Autodesk Inventor part; units mm, degrees
ref_plane "Work Plane3" through (1.5, 0, 13) normal (1, 0, 0) x (0, 0, -1)
ref_plane "Work Plane5" through (3, 0, 0) normal (0, 0, 1) x (0, 1, 0)
ref_plane "Work Plane6" through (0, 1.1, 0) normal (0, -1, 0) x (1, 0, 0)
sketch "Sketch1" plane through (0, 0, 0) normal (0, 1, 0) x (-1, 0, 0)
  line L0 (0, 0) -> (0, -5)
  line L1 (0, 0) -> (0, 5)
  line L2 (0, 5) -> (-3, 5)
  line L3 (0, -5) -> (-3, -5)
  line L4 (-3, 5) -> (-3, 13)
  line L5 (-3, -5) -> (-3, -13)
  line L6 (1.5, 0) -> (1.5, -5)
  line L7 (1.5, 0) -> (1.5, 5)
  spline S0 degree 3 poles (-3, 13) (1.5, 11.5121) (1.5, 8.2561) (1.5, 5) knots 0 0 0 0 1 1 1 1
  spline S1 degree 3 poles (-3, -13) (1.5, -11.5121) (1.5, -8.2561) (1.5, -5) knots 0 0 0 0 1 1 1 1
  point P0 (-3, 9)
  point P1 (-3, -9)
  dimension "d0" = 5
  dimension "d1" = 5
  dimension "d2" = 3
  dimension "d3" = 3
  dimension "d4" = 8
  dimension "d5" = 8
  dimension "d6" = 5
  dimension "d7" = 5
extrude "Extrusion1" add sketch "Sketch1" along normal blind 5
sketch "Sketch2" plane through (3, 0, 13) normal (1, 0, 0) x (0, 0, -1)
  circle A0 centre (3.5513, 2.5007) radius 1
  line L0 (13, 0) -> (13, 5)
  line L1 (8, 5) -> (18, 5)
  line L2 (4.7093, 4.4988) -> (5.8606, 2.4969)
  line L3 (5.8606, 2.4969) -> (4.7026, 0.4988)
  line L4 (4.7026, 0.4988) -> (2.3933, 0.5026)
  line L5 (2.3933, 0.5026) -> (1.2419, 2.5045)
  line L6 (1.2419, 2.5045) -> (2.3999, 4.5026)
  line L7 (2.3999, 4.5026) -> (4.7093, 4.4988)
  point P0 (22, 2.5)
  dimension "d12" = 2
  dimension "d33" = 4
extrude "Extrusion2" cut sketch "Sketch2" against normal blind 2 contours A0
ref_plane "Work Plane3" through (1.5, 0, 13) normal (1, 0, 0) x (0, 0, -1)
sketch "Sketch3" plane through (1.5, 0, 13) normal (1, 0, 0) x (0, 0, -1)
  circle A0 centre (3.5513, 2.5007) radius 1
  circle A1 centre (3.5513, 2.5007) radius 1
  line L0 (0, 0) -> (8, 0)
  line L1 (8, 0) -> (8, 5)
  line L2 (0, 5) -> (8, 5)
  line L3 (0, 0) -> (0, 5)
  line L4 (2.3935, 0.5024) -> (1.2419, 2.5042)
  line L5 (1.2419, 2.5042) -> (2.3996, 4.5024)
  line L6 (2.3996, 4.5024) -> (4.709, 4.4989)
  line L7 (4.709, 4.4989) -> (5.8607, 2.4972)
  line L8 (5.8607, 2.4972) -> (4.7029, 0.4989)
  line L9 (4.7029, 0.4989) -> (2.3935, 0.5024)
  circle A2 centre (3.5513, 2.5007) radius 1
  point P0 (13, 0)
extrude "Extrusion3" cut sketch "Sketch3" against normal blind 10 contours A0 | L4 L5 L6 L7 L8 L9
ref_plane "Work Plane5" through (3, 0, 0) normal (0, 0, 1) x (0, 1, 0)
mirror "Mirror1" about plane through (3, 0, 0) normal (0, 0, 1) of "Extrusion2", "Extrusion3"
ref_plane "Work Plane6" through (0, 1.1, 0) normal (0, -1, 0) x (1, 0, 0)
sketch "Sketch5" plane through (0, 1.1, 0) normal (0, -1, 0) x (1, 0, 0)
  line L0 (3, 5) -> (0, 5)
  line L1 (0, 5) -> (0, -5)
  line L2 (1, 5) -> (0, 4)
  line L3 (0, -5) -> (3, -5)
  line L4 (1, -5) -> (0, -4)
  point P0 (0, 0)
extrude "Extrusion4" add sketch "Sketch5" against normal blind 0.5
ref_plane "Work Plane7" through (0, 4.9, 0) normal (0, 1, 0) x (1, 0, 0)
sketch "Sketch6" plane through (0, 4.9, 0) normal (0, 1, 0) x (1, 0, 0)
  line L0 (1, -5) -> (0, -5)
  line L1 (1, -5) -> (0, -4)
  line L2 (0, -5) -> (0, -4)
  line L3 (0, 4) -> (0, 5)
  line L4 (0, 4) -> (1, 5)
  line L5 (0, 5) -> (1, 5)
  point P0 (0, 0)
extrude "Extrusion5" add sketch "Sketch6" against normal blind 0.5
properties part number "top_mount"
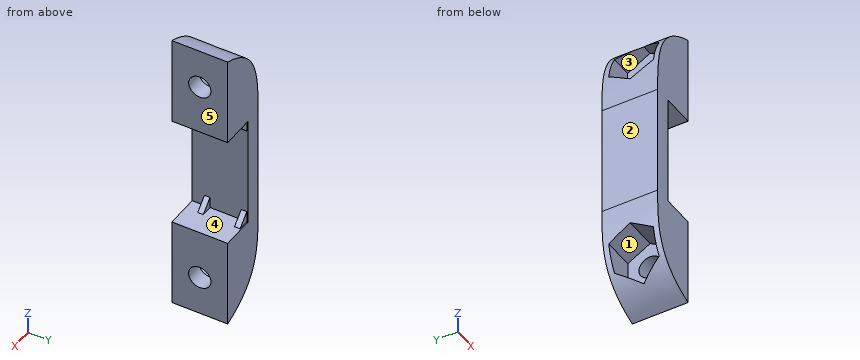
Can you work these out from the model? Positions are in its coordinate system, mm. Face numbers are marked on the shaded views. A direction names the side the tool comes from. Round coordinates to 2 decimals unless told otherwise and drop trailing zeros. Order: outer loops, then holes, each group sorted by start corner. A loop starts at its lowest first (then second) coordinate and runs counter-clockwise, first axis right, second up.
(1) If we section it at A-A (z = 2.25): Please give me the cut outline in (x, y).
Results are:
outline: (-1.5, 0) - (0, 0) - (0, 5) - (-1.5, 5) - close
(2) We'd pull the mould along Z, two halves only. Please class the marked faces 1 and 2: +Z half, -Z half, draft (parallel to the pull), parting line (faces both ways), or undercut.
Results are:
face 1: undercut
face 2: draft
(3) I'm going to push flat-ended pins straight in: pin 1 (2.5 mm diameter, centred on y = 3.5, z = 0, fed in from +X); pin 2 (1.5 mm diameter, centred on x = 2, y = 1.5, fed in from +Z); pin 3 (1.5 mm diameter, centred on y = 2, z = -8, fed in from -X). Where does each tip first touch, or does it pass through?
Results are:
pin 1: stops at x = 0
pin 2: stops at z = 12.91
pin 3: stops at x = -1.44
(4) If I drill on L1, parallel to Z at x = 2.45, y = 2; L2, parallel to Y at x = -0.45, z = 8.75; L3, parallel to Z at x = 1.25, y = 2.05, over which ranges is the centre line in solid material (lowest first)?
Results are:
L1: z = -12.8 to -10.31, -8.58 to -5, 5 to 8.58, 10.31 to 12.8
L2: y = 0 to 0.5, 4.5 to 5
L3: z = -12.21 to -11.5, -7.4 to -5, 5 to 7.4, 11.5 to 12.21
(5) On a 3-axis mill with a long thin cutter (end or side, diameter ignored), from which of +Z, -Z, +X, -X, +Y, -Y can I reach the whole of each face in a straight line? I mean the marked faces 3, 4 and 5. Say none if no direction works.
Results are:
face 3: -X
face 4: +X
face 5: +Z, -Z, +X, +Y, -Y
(6) If we section it at B-B (y = 2.25): Count the separate pieces of the cut face and the enclosed holes in it, plus the area to 3 significant figures.
Results are:
separate pieces: 3
enclosed holes: 0
area: 46.8 mm2
